Read the model definition and answer for the solid it produces. Units are mm, in the model's axes. A direction names the side the tool comes from. Coordinates: 2 decimals unless noted, no trailing zeros. Order: outer loops, then holes, each group sorted by start corner. A loop starts at its lowest first (then second) coordinate and runs counter-clockwise, first axis right, second up. Notation, with made-up numbers: M 74,-2 L 94,-2 A8 ccw 94,12 Z; hole C 69.25,-8 d5. An arc over 180 degrees is marked long. One line per question, with ' | ' between items. Start each with the question number.
1) Find section B-B, the plane x = 6.35. Write down the section's boundary in (y, z), plus the area to 3 significant figures.
2) Given P1, Ø2, axis at x = 4.49, y = -4.49, coming from the -Z side; P2, Ø2, axis at x = -7, y = 3.5, coming from the +Z side; P3, Ø8, axis at x = -1.5, y = -2, coming from the -Z side; P4, Ø10, axis at x = -5, y = 4, coming from the +Z side, each flat-ended and moving along its own axis, determine where each tip first touches the part or whether it passes through.
3) Find section C-C, the plane x = 0.25. Write down the section's boundary in (y, z), plus the area to 3 significant figures.
4) A tool of negligible diameter and unlimited length cuts with its end or side. For faces 1 (the face through (0.43, 9.44, -0.99)), 2 (the face through (1.65, -0.69, 0.41)), from which of +Z, -Z, +X, -X, +Y, -Y can it reach the whole face along a straight path? Write none if from no direction.
5) Consider probe 1 along X at (y, z) = (0.5, -1.95); probe 2 along X at (y, z) = (-8.75, -1.75); probe 3 along X at (y, z) = (-6, -0.4). Determine where each line is inside the solid, lowest interval first.
6) Find section D-D, the plane z = 1.05. Write down the section's boundary in (x, y), plus the area to 3 significant figures.
7) The mould has two halves that part along Y. Classify faces 3 (the face through (4.856, -5.194, -0.986)), 4 (the face through (0, 0, -3)), 5 (the face through (2.1, 0.66, -2.49)): +Y half, -Y half, draft (parallel to the pull), parting line (faces both ways), or undercut.
8) Find section A-A, the plane y = 0. Write down the section's boundary in (x, z), plus the area to 3 significant figures.
from build123d import *

# Parameters (mm, degrees)
F0_W     = 1.7891867319
F0_H     = 0.8
F2_R     = 0.79375
F3_DEPTH = 25.4


with BuildPart() as f1:
    # F0 (on Front) → F1 (revolve)
    with BuildSketch(Plane.XZ):
        with Locations((0.894593366, 0.4)):
            Rectangle(F0_W, F0_H)
        Polygon((1.7891867319, 0), (0, 0), (0, -3), (2.2, -3), (2.2, -2), (10, -2), (10, 0), align=None)
    revolve(axis=Axis((0, 0, -1.5), (0, 0, 1)))

    # F2 (on face) → F3 (cut)
    with BuildSketch(Plane.XY):
        with BuildLine():
            ThreePointArc((0.79375, 6.35), (-0.5612660076, 6.9112660076), (0, 5.55625))
            ThreePointArc((0, 5.55625), (0.5612660076, 5.7887339924), (0.79375, 6.35))
        make_face()
        with BuildLine():
            Line((2.4300397955, 5.8666350314), (2.1262848211, 5.1333056525))
            ThreePointArc((2.1262848211, 5.1333056525), (2.871023668, 5.2066560267), (3.2237897955, 5.8666350314))
            ThreePointArc((3.2237897955, 5.8666350314), (3.0900188003, 6.3076189039), (2.73379477, 6.5999644104))
            Line((2.73379477, 6.5999644104), (2.4300397955, 5.8666350314))
        make_face()
        with BuildLine():
            ThreePointArc((2.73379477, 6.5999644104), (1.6967104166, 6.1703900059), (2.1262848211, 5.1333056525))
            Line((2.1262848211, 5.1333056525), (2.4300397955, 5.8666350314))
            Line((2.4300397955, 5.8666350314), (2.73379477, 6.5999644104))
        make_face()
        with BuildLine():
            Line((4.4901280605, 4.4901280605), (3.928862053, 3.928862053))
            ThreePointArc((3.928862053, 3.928862053), (4.793883035, 3.7567986816), (5.2838780605, 4.4901280605))
            ThreePointArc((5.2838780605, 4.4901280605), (5.2234574395, 4.793883035), (5.0513940681, 5.0513940681))
            Line((5.0513940681, 5.0513940681), (4.4901280605, 4.4901280605))
        make_face()
        with BuildLine():
            ThreePointArc((5.0513940681, 5.0513940681), (3.928862053, 5.0513940681), (3.928862053, 3.928862053))
            Line((3.928862053, 3.928862053), (4.4901280605, 4.4901280605))
            Line((4.4901280605, 4.4901280605), (5.0513940681, 5.0513940681))
        make_face()
        with BuildLine():
            ThreePointArc((3.6618567991, 8.8405043479), (2.6247724457, 8.4109299434), (3.0543468502, 7.37384559))
            Line((3.0543468502, 7.37384559), (3.6618567991, 8.8405043479))
        make_face()
        with BuildLine():
            Line((3.6618567991, 8.8405043479), (3.0543468502, 7.37384559))
            ThreePointArc((3.0543468502, 7.37384559), (3.7990856971, 7.4471959642), (4.1518518247, 8.107174969))
            ThreePointArc((4.1518518247, 8.107174969), (4.0180808294, 8.5481588414), (3.6618567991, 8.8405043479))
        make_face()
        with BuildLine():
            ThreePointArc((6.7662290954, 6.7662290954), (5.6436970802, 6.7662290954), (5.6436970802, 5.6436970802))
            Line((5.6436970802, 5.6436970802), (6.7662290954, 6.7662290954))
        make_face()
        with BuildLine():
            Line((6.7662290954, 6.7662290954), (5.6436970802, 5.6436970802))
            ThreePointArc((5.6436970802, 5.6436970802), (6.5087180622, 5.4716337089), (6.9987130878, 6.2049630878))
            ThreePointArc((6.9987130878, 6.2049630878), (6.9382924667, 6.5087180622), (6.7662290954, 6.7662290954))
        make_face()
        with Locations((-6.35, 0)):
            Circle(F2_R)
        with Locations((-5.8666350314, 2.4300397955)):
            Circle(F2_R)
        with Locations((-4.4901280605, 4.4901280605)):
            Circle(F2_R)
        with Locations((0, -6.35)):
            Circle(F2_R)
        with Locations((-2.4300397955, -5.8666350314)):
            Circle(F2_R)
        with Locations((-4.4901280605, -4.4901280605)):
            Circle(F2_R)
        with Locations((6.35, 0)):
            Circle(F2_R)
        with Locations((5.8666350314, -2.4300397955)):
            Circle(F2_R)
        with Locations((4.4901280605, -4.4901280605)):
            Circle(F2_R)
        with Locations((0, 8.7751429528)):
            Circle(F2_R)
        with Locations((0, -8.7751429528)):
            Circle(F2_R)
        with Locations((-3.3581018247, -8.107174969)):
            Circle(F2_R)
        with Locations((-6.2049630878, -6.2049630878)):
            Circle(F2_R)
    extrude(amount=-F3_DEPTH, mode=Mode.SUBTRACT)

    # F4 (on Front) → F5 (revolve)
    with BuildSketch(Plane.XZ):
        with BuildLine():
            Line((-1.7891867319, 0.8), (0, 0.8))
            Line((0, 0.8), (0, 1.5092346721))
            ThreePointArc((0, 1.5092346721), (-0.9623153046, 1.3254595112), (-1.7891867319, 0.8))
        make_face()
    revolve(axis=Axis((0, 0, 1.1546173361), (0, 0, 1)))


solid = f1.part
Report:
1) outline: M -7.73,-2 L -3.06,-2 L -3.06,0 L -7.73,0 Z; M -1.8,-2 L -0.79,-2 L -0.79,0 L -1.8,0 Z; M 0.79,-2 L 5.42,-2 L 5.42,0 L 0.79,0 Z; M 6.99,-2 L 7.73,-2 L 7.73,0 L 6.99,0 Z | area: 22.1 mm^2
2) P1: stops at z = -2 | P2: stops at z = 0 | P3: stops at z = -3 | P4: stops at z = 1.1
3) outline: M -10,-2 L -9.53,-2 L -9.53,0 L -10,0 Z; M -8.02,-2 L -7.1,-2 L -7.1,0 L -8.02,0 Z; M -5.6,-2 L -2.19,-2 L -2.19,-3 L 2.19,-3 L 2.19,-2 L 5.6,-2 L 5.6,0 L 1.77,0 L 1.77,0.8 A2.6 ccw -1.77,0.8 L -1.77,0 L -5.6,0 Z; M 7.1,-2 L 8.02,-2 L 8.02,0 L 7.1,0 Z; M 9.53,-2 L 10,-2 L 10,0 L 9.53,0 Z | area: 36.8 mm^2
4) face 1: +Z, -Z | face 2: +Z
5) probe 1: x = -9.99 to -6.97, -5.73 to 5.73, 6.97 to 9.99 | probe 2: x = -4.84 to -3.82, -2.89 to -0.79, 0.79 to 4.84 | probe 3: x = -8 to -6.97, -5.44 to -3.21, -1.65 to -0.71, 0.71 to 8
6) outline: C 0,0 d2.96 | area: 6.87 mm^2
7) face 3: undercut | face 4: draft | face 5: parting line
8) outline: M -10,-2 L -7.14,-2 L -7.14,0 L -10,0 Z; M -5.56,-2 L -2.2,-2 L -2.2,-3 L 2.2,-3 L 2.2,-2 L 5.56,-2 L 5.56,0 L 1.79,0 L 1.79,0.8 A2.61 ccw -1.79,0.8 L -1.79,0 L -5.56,0 Z; M 7.14,-2 L 10,-2 L 10,0 L 7.14,0 Z | area: 42.7 mm^2
